Print and shaded views of the part. All mm, measured from the part's lowest x, y and z. A direction names the side the tool comes from. Coordinates: 2 decimals unless noted, no trailing zeros. Order: outer loops, then holes, each group sorted by start corner. A loop starts at its lowest first (then second) coordinate and runs counter-clockwise, first axis right, second up. Notation, with made-up numbers: M 48.25,-31.5 L 58.25,-31.5 A29 ccw 58.25,-8.5 Z; hole C 51.5,85.25 d6. An arc over 180 degrees is marked long. Return JSON: item names as keys, results as strings.
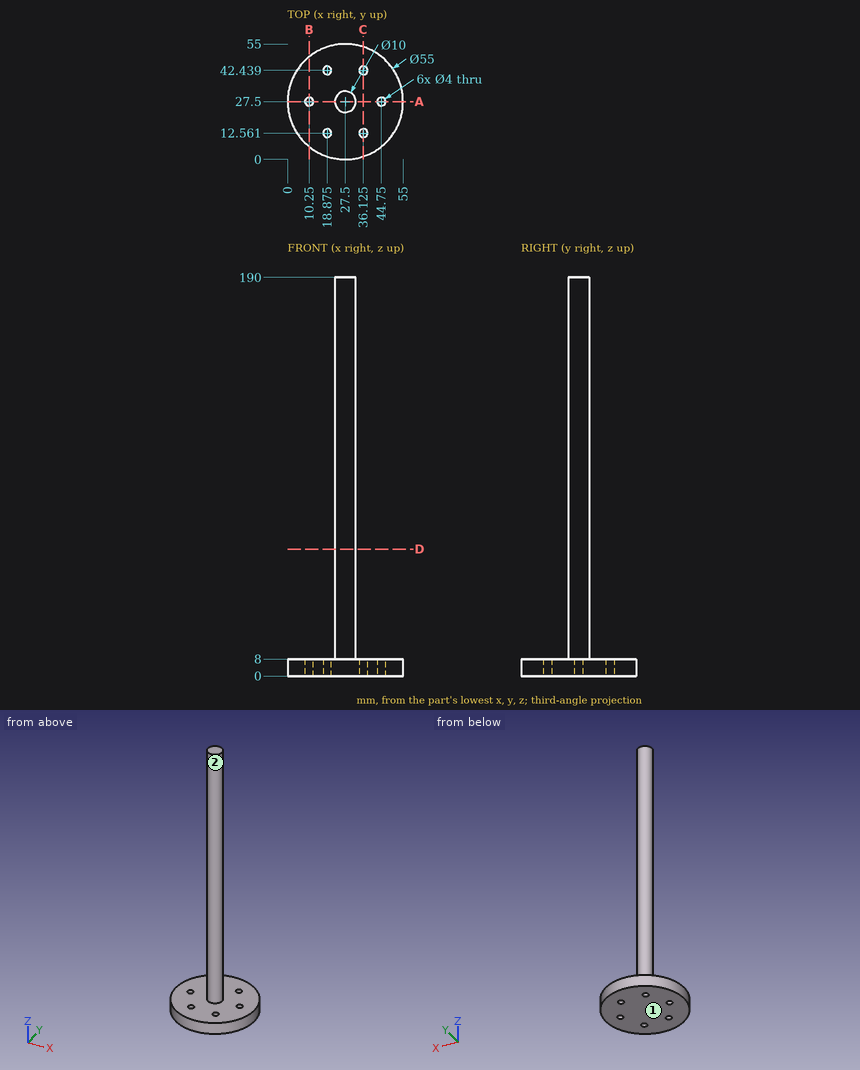
Item 1: Drop flat-ended pins along their axis: pin 1 Ø10 at (x, z) = (20.5, 42.5) entering from -Y; pin 2 Ø10 at (y, z) = (31, 56) entering from -X; pin 3 Ø5 at (x, y) = (36.12, 12.56) entering from +Z. Give the stop position or say it passes through.
Check result:
{"pin 1": "stops at y = 22.92", "pin 2": "stops at x = 22.5", "pin 3": "stops at z = 8"}
Item 2: Saw through at C-C (x = 36). Write the cut outline in (y, z) (1 decimal), and give its area (3 significant figures).
Check result:
{"outline": "M 1.3,0 L 10.6,0 L 10.6,8 L 1.3,8 Z; M 14.6,0 L 40.4,0 L 40.4,8 L 14.6,8 Z; M 44.4,0 L 53.7,0 L 53.7,8 L 44.4,8 Z", "area": "355 mm2"}
Item 3: Saw through at A-A (y = 27.5). Write the cut outline in (x, z), and give its area (3 significant figures).
Check result:
{"outline": "M 0,0 L 8.25,0 L 8.25,8 L 0,8 Z; M 12.25,0 L 42.75,0 L 42.75,8 L 32.5,8 L 32.5,190 L 22.5,190 L 22.5,8 L 12.25,8 Z; M 46.75,0 L 55,0 L 55,8 L 46.75,8 Z", "area": "2,200 mm2"}
Item 4: Wall check: line 1 (X direction, y = 27, z = 5); line 2 (Z direction, x = 24, y = 17); line 3 (Y direction, x = 44.75, z = 5.5). Give the ranges that are in metal, low to high.
Check result:
{"line 1": "x = 0 to 8.31, 12.19 to 42.81, 46.69 to 55", "line 2": "z = 0 to 8", "line 3": "y = 6.08 to 25.5, 29.5 to 48.92"}
Item 5: 3-axis set-ups, long thin cutter, end or side, ignore diameter. For the marked faces 1 and 2: which of +Z, -Z, +X, -X, +Y, -Y reach the whole face in a straight line?
Check result:
{"face 1": "-Z, +X, -X, +Y, -Y", "face 2": "+Z"}
Item 6: Saw through at B-B (x = 10.25). Write the cut outline in (y, z), and give its area (3 significant figures).
Check result:
{"outline": "M 6.08,0 L 25.5,0 L 25.5,8 L 6.08,8 Z; M 29.5,0 L 48.92,0 L 48.92,8 L 29.5,8 Z", "area": "311 mm2"}
Item 7: Saw through at D-D (z = 60.5). Write the cut outline in (x, y), and give its area (3 significant figures).
Check result:
{"outline": "C 27.5,27.5 d10", "area": "78.5 mm2"}
